```python
from build123d import *

# Parameters (mm, degrees)
SKETCH_R              = 6.5
SKETCH_R_2            = 2.5
PAD_DEPTH             = 13
SKETCH001_R           = 1.5
POCKET_DEPTH          = 20
POLARPATTERN_COUNT    = 6
SKETCH002_R           = 2.75
POCKET001_DEPTH       = 3
POLARPATTERN001_COUNT = 6
POCKET002_DEPTH       = 5


with BuildPart() as part:
    # Sketch → Pad (new body)
    with BuildSketch(Plane.XY):
        with BuildLine():
            ThreePointArc((25.617377, 10), (-27.5, 0), (25.617377, -10))
            Line((25.617377, -10), (35, -10))
            ThreePointArc((35, -10), (45, 0), (35, 10))
            Line((25.617377, 10), (35, 10))
        make_face()
        Circle(SKETCH_R, mode=Mode.SUBTRACT)
        with Locations((35, 0)):
            Circle(SKETCH_R_2, mode=Mode.SUBTRACT)
    extrude(amount=PAD_DEPTH)

    # Sketch001 (on Face8 of Pad) → Pocket (cut)
    with BuildSketch(Plane.XY.offset(13)):
        with Locations((22, 0)):
            Circle(SKETCH001_R)
    pocket = extrude(amount=-POCKET_DEPTH, mode=Mode.SUBTRACT)

    # PolarPattern: Pocket ×6 about axis
    polarpattern_axis = Axis((0, 0, 13), (0, 0, 1))
    for i in range(1, POLARPATTERN_COUNT):
        add(pocket.rotate(polarpattern_axis, i * 360 / POLARPATTERN_COUNT), mode=Mode.SUBTRACT)

    # Sketch002 (on Face5 of PolarPattern) → Pocket001 (cut)
    with BuildSketch(Plane.XY.offset(13)):
        with Locations((22, 0)):
            Circle(SKETCH002_R)
    pocket001 = extrude(amount=-POCKET001_DEPTH, mode=Mode.SUBTRACT)

    # PolarPattern001: Pocket001 ×6 about axis
    polarpattern001_axis = Axis((0, 0, 13), (0, 0, 1))
    for i in range(1, POLARPATTERN001_COUNT):
        add(pocket001.rotate(polarpattern001_axis, i * 360 / POLARPATTERN001_COUNT), mode=Mode.SUBTRACT)

    # Sketch003 (on Face4 of PolarPattern001) → Pocket002 (cut)
    with BuildSketch(Plane(origin=(0, 0, 0), x_dir=(1, 0, 0), z_dir=(0, 0, -1))):
        Polygon((39.503332, 0), (37.251666, 3.9), (32.748334, 3.9), (30.496668, 0), (32.748334, -3.9), (37.251666, -3.9), align=None)
    extrude(amount=-POCKET002_DEPTH, mode=Mode.SUBTRACT)


solid = part.part
```
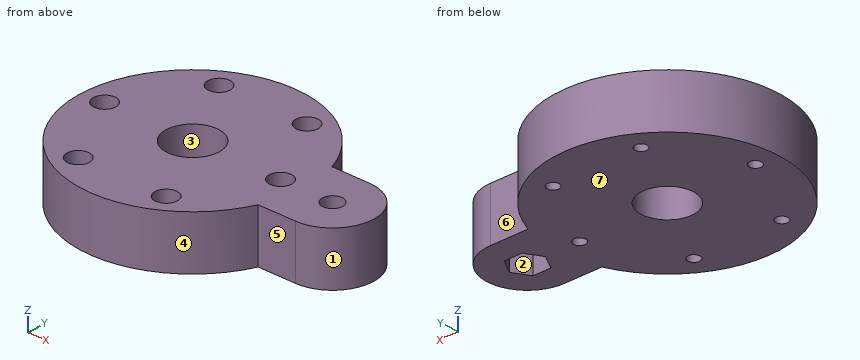
Geometry: final body of the model. Coordinates: model frame, mm. Face numbers are marked on the shaded views. A direction names the side the tool comes from. Round coordinates to 2 decimals unless told otherwise and drop trailing zeros. Order: outer loops, then holes, each group sorted by start corner. A loop starts at its lowest first (then second) coordinate and runs counter-clockwise, first axis right, second up. Notation, with made-up numbers: M 69,56 L 123,56 A21 ccw 123,67 Z; hole C 70.5,72 d11. An arc over 180 degrees is marked long. Use one line per item in the form item = value. Start each with the question number.
Q1. Cut plane D-D (y = 11.5). Return loops of the section in (x, z), and give its area (3 significant figures).
Q2. Mould query, pull axis X, two halves, no side actions, for the marked faces 1, 2, 3 and 4. Classes: +X half, -X half, draft (parallel to the pull), parting line (faces both ways), or undercut.
Q3. Cut plane A-A (x = 0). Return loops of the section in (y, z).
Q4. Pin query (flat end, axial travel): pin 1 Ø1 at (x, z) = (8, 11.5) entering from -Y; pin 2 Ø4 at (x, z) = (14.5, 2.5) entering from +Y; pin 3 Ø5 at (x, z) = (4.5, 5) entering from +Y; pin 4 Ø11.5 at (x, y) = (0, 0) entering from +Z. Return the tip coordinate at first contact, or that it passes through.
Q5. Access query for the marked faces 5, 6 and 7. Directions: +Z, -Z, +X, -X, +Y, -Y. A direction counts if a zero-diameter tool reaches every point of the face in a straight line with its end or side. Return the directions, or none.
Q6. Cut plane C-C (z = 8). Count the separate pieces of the cut face and the enclosed holes in it, and give its area (3 significant figures).
Q7. Cut plane B-B (x = 11). Return loops of the section in (y, z), and give its area (3 significant figures).
Q8. Material intervals for line 1 (Y direction, x = 11, z = 8); line 2 (X direction, y = 18, z = 4.75); line 3 (Y direction, x = -11, z = 11.75), sorted ascending. Write a range as [from, to].
Geometry results:
q1.outline = M -24.98,0 L 24.98,0 L 24.98,13 L -24.98,13 Z
q1.area = 649 mm^2
q2.face_1 = +X half
q2.face_2 = undercut
q2.face_3 = undercut
q2.face_4 = parting line
q3.outline = M -27.5,0 L -6.5,0 L -6.5,13 L -27.5,13 Z; M 6.5,0 L 27.5,0 L 27.5,13 L 6.5,13 Z
q4.pin_1 = -26.46
q4.pin_2 = 24.49
q4.pin_3 = 27.43
q4.pin_4 = through
q5.face_5 = +Z, -Z, +X, -Y
q5.face_6 = +Z, -Z, +X, +Y
q5.face_7 = -Z, +X, -X, +Y, -Y
q6.separate_pieces = 1
q6.enclosed_holes = 8
q6.area = 2,500 mm^2
q7.outline = M -25.2,0 L -20.55,0 L -20.55,10 L -21.8,10 L -21.8,13 L -25.2,13 Z; M -17.55,0 L 17.55,0 L 17.55,10 L 16.3,10 L 16.3,13 L -16.3,13 L -16.3,10 L -17.55,10 Z; M 20.55,0 L 25.2,0 L 25.2,13 L 21.8,13 L 21.8,10 L 20.55,10 Z
q7.area = 562 mm^2
q8.line_1 = [-25.2, -20.55], [-17.55, 17.55], [20.55, 25.2]
q8.line_2 = [-20.79, -12.07], [-9.93, 9.93], [12.07, 20.79]
q8.line_3 = [-25.2, -21.8], [-16.3, 16.3], [21.8, 25.2]
